Geometry check sheet. Reference: the model listing, model coordinates, mm. Face numbers are marked on the shaded views. Coordinates: 2 decimals unless noted, no trailing zeros. Order: outer loops, then holes, each group sorted by start corner. A loop starts at its lowest first (then second) coordinate and runs counter-clockwise, first axis right, second up. Notation, with made-up numbers: M 36,-26 L 87,-26 A15 cw 87,1 Z; hole C 87.5,62 d9. An arc over 180 degrees is marked long. Use CSV: the item, a comma, the result in double quotes. Start each with the question number.
```python
from build123d import *

# Parameters (mm, degrees)
F0_W     = 101.6
F0_H     = 139.7
F1_DEPTH = 25.4
F3_D     = 8.4328
F3_DEPTH = 25.4
F3_TIP   = 2.5334687141
F4_R     = 20.6121
F5_DEPTH = 9.525
F6_R     = 15.875
F7_DEPTH = 25.4


with BuildPart() as f1:
    # F0 (on Front) → F1 (new body)
    with BuildSketch(Plane.XZ):
        with Locations((9.0106602939, -2.4217218161)):
            Rectangle(F0_W, F0_H)
    extrude(amount=F1_DEPTH)

    # F3
    with Locations(Plane(origin=(0, 0, -72.2717218161), x_dir=(1, 0, 0), z_dir=(0, 0, -1))):
        with Locations((-16.3893397061, 12.7), (34.4106602939, 12.7)):
            Hole(F3_D / 2, depth=F3_DEPTH)
            with Locations((0, 0, -(F3_DEPTH + F3_TIP / 2))):  # 118° drill point
                Cone(0, F3_D / 2, F3_TIP, mode=Mode.SUBTRACT)

    # F4 (on face) → F5 (cut)
    with BuildSketch(Plane.XZ.offset(25.4)):
        with Locations((9.0106602939, 16.6282781839)):
            Circle(F4_R)
    extrude(amount=-F5_DEPTH, mode=Mode.SUBTRACT)

    # F6 (on face) → F7 (cut)
    with BuildSketch(Plane.XZ.offset(15.875)):
        with Locations((9.0106602939, 16.6282781839)):
            Circle(F6_R)
    extrude(amount=-F7_DEPTH, mode=Mode.SUBTRACT)


solid = f1.part
```
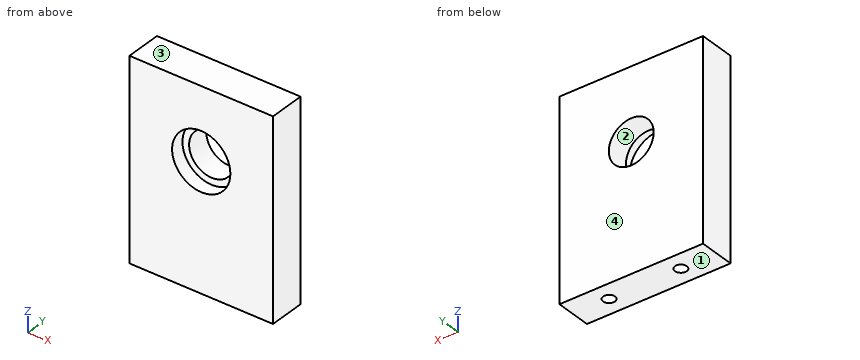
1) Section check D-D on z = -55.5. Record the boundary of the cut face in (x, y).
2) Draft check along Z on the marked faces 1, 2, 3 and 4. Enter one of: +Z half, -Z half, draft (parallel to the pull), parting line (faces both ways), or undercut.
3) Section check C-C on y = -2. Record the boundary of the cut face in (x, z) (3 decimals), then the cut area to 3 significant figures.
4) Material ranges on line 1 along X through (y, z) = (-22, 30); line 2 along Z through (x, y) = (13.5, -11.75); line 3 along Y through (x, z) = (29.5, 15) (3 decimals), recorded low to high.
5) Section check B-B on z = 10. Record the boundary of the cut face in (x, y) (3 decimals).
6) Section check A-A on x = 9. Record the boundary of the cut face in (y, z) (3 decimals), then the cut area to 3 significant figures.
Results are:
1,outline,"M -41.79,-25.4 L 59.81,-25.4 L 59.81,0 L -41.79,0 Z; hole C -16.39,-12.7 d8.43; hole C 34.41,-12.7 d8.43"
2,face 1,"-Z half"
2,face 2,"undercut"
2,face 3,"+Z half"
2,face 4,"draft"
3,outline,"M -41.789,-72.272 L 59.811,-72.272 L 59.811,67.428 L -41.789,67.428 Z; hole C 9.011,16.628 d31.75"
3,area,"13,400 mm²"
4,line 1,"x = -41.79 to -6.68, 24.7 to 59.81"
4,line 2,"z = -72.27 to 1.4, 31.86 to 67.43"
4,line 3,"y = -15.875 to 0"
5,outline,"M -41.789,-25.4 L -10.507,-25.4 L -10.507,-15.875 L -5.414,-15.875 L -5.414,0 L -41.789,0 Z; M 23.436,-15.875 L 28.528,-15.875 L 28.528,-25.4 L 59.811,-25.4 L 59.811,0 L 23.436,0 Z"
6,outline,"M -25.4,-72.272 L 0,-72.272 L 0,0.753 L -15.875,0.753 L -15.875,-3.984 L -25.4,-3.984 Z; M -25.4,37.24 L -15.875,37.24 L -15.875,32.503 L 0,32.503 L 0,67.428 L -25.4,67.428 Z"
6,area,"2,650 mm²"
